from build123d import *

# Parameters (mm, degrees)
BOSS_EXTRU_1_DEPTH      = 30
ENL_V_MAT_EXTRU_1_DEPTH = 24.3
ESQUISSE5_W             = 3.7
ESQUISSE5_H             = 3.7
BOSS_EXTRU_5_DEPTH      = 24.3


with BuildPart() as part:
    # Esquisse1 → Boss.-Extru.1 (new body)
    with BuildSketch(Plane(origin=(0, 0, 0), x_dir=(1, 0, 0), z_dir=(0, 1, 0))):
        Polygon((0, 0), (0, -15), (35, -15), (35, -50), (50, -50), (50, 0), align=None)
    extrude(amount=BOSS_EXTRU_1_DEPTH)

    # Esquisse2 → Enlèv. mat.-Extru.1 (cut)
    with BuildSketch(Plane.XZ):
        Polygon((40.7, 50), (40.7, 9.3), (0, 9.3), (0, 5.7), (44.3, 5.7), (44.3, 50), align=None)
    extrude(amount=-ENL_V_MAT_EXTRU_1_DEPTH, mode=Mode.SUBTRACT)

    # Esquisse5 → Boss.-Extru.5 (add)
    with BuildSketch(Plane.XZ.offset(-24.3)):
        with Locations((42.45, 7.55)):
            Rectangle(ESQUISSE5_W, ESQUISSE5_H)
    extrude(amount=BOSS_EXTRU_5_DEPTH)


solid = part.part
Build history of the part. All positions in model axes, mm. A direction names the side the tool comes from. Round coordinates to 2 decimals unless told otherwise and drop trailing zeros. Write each loop counter-clockwise with the first axis right and the second up, starting at its lowest first coordinate (ties: lowest second). Pieces come first, ordered by that corner, then holes. Notation, with made-up numbers: (16, 22.5) -> (35, 22.5) arc R25 cw to (35, 38.5) -> close; hole circle Ø5 at (40, -32). An arc over 180 degrees is marked (long way). Write item = value, one per line.
(1) Band-saw the part on D-D (y = 27.5). Give the cut face in (x, z), then the cut area to 4 significant figures.
Answer:
outline = (0, 0) -> (50, 0) -> (50, 50) -> (35, 50) -> (35, 15) -> (0, 15) -> close
area = 1,275 mm2
(2) Band-saw the part on A-A (x = 4). Give the cut face in (y, z), then the cut area to 3 significant figures.
Answer:
outline = (0, 0) -> (30, 0) -> (30, 15) -> (0, 15) -> (0, 9.3) -> (24.3, 9.3) -> (24.3, 5.7) -> (0, 5.7) -> close
area = 363 mm2
(3) Probe L1, parallel to X at y = 2.25, z = 34; L2, parallel to Z at x = 27.5, y = 22; L3, parallel to X at y = 7.5, z = 10. List the from-to ranges inside material, lowest first.
Answer:
L1 = 35 to 40.7, 44.3 to 50
L2 = 0 to 5.7, 9.3 to 15
L3 = 0 to 40.7, 44.3 to 50
(4) Tool access for faces 1 (the face through (44.3, 12, 29)), 2 (the face through (17, 15, 15)), 3 (the face through (25, 15, 0)), 4 (the face through (20, 12, 5.7)): list every direction of +Z, -Z, +X, -X, +Y, -Y with a clear straight run to the whole face (end or side of a thin tool).
Answer:
face_1 = +Z, -Y
face_2 = +Z, -X, +Y, -Y
face_3 = -Z, +X, -X, +Y, -Y
face_4 = -X, -Y
(5) Two-plate mould, pull along X, no slides. Class faces 5 (the face through (40.7, 12, 30)), 6 (the face through (21, 12, 9.3)), 7 (the face through (35, 15, 32)): pulls with the +X half, pulls with the -X half, needs draft (parallel to the pull), parting line crosses it, or undercut.
Answer:
face_5 = undercut
face_6 = needs draft
face_7 = pulls with the -X half
(6) Band-saw the part on C-C (z = 37). Give the cut face in (x, y).
Answer:
outline = (35, 0) -> (40.7, 0) -> (40.7, 24.3) -> (44.3, 24.3) -> (44.3, 0) -> (50, 0) -> (50, 30) -> (35, 30) -> close
(7) Flat gauge pins, fed straight in: pin 1 (2 mm diameter, centred on x = 26, y = 19.5, fed in from +Z); pin 2 (3 mm diameter, centred on x = 42.5, z = 34, fed in from -Y); pin 3 (12 mm diameter, centred on y = 15.5, z = 24.5, fed in from -X). Where does each tip first touch, or does it go through?
Answer:
pin_1 = 15
pin_2 = 24.3
pin_3 = 35
(8) Band-saw the part on B-B (y = 5.25). Give the cut face in (x, z).
Answer:
outline = (0, 0) -> (50, 0) -> (50, 50) -> (44.3, 50) -> (44.3, 9.4) -> (40.7, 9.4) -> (40.7, 50) -> (35, 50) -> (35, 15) -> (0, 15) -> (0, 9.3) -> (40.6, 9.3) -> (40.6, 5.7) -> (0, 5.7) -> close
